Here's how the part is built. I have some questions about the finished solid (model axes, mm). Face numbers are marked on the shaded views. A direction names the side the tool comes from. Round coordinates to 2 decimals unless told otherwise and drop trailing zeros. Order: outer loops, then holes, each group sorted by start corner. A loop starts at its lowest first (then second) coordinate and runs counter-clockwise, first axis right, second up. Notation, with made-up numbers: (80, -20) - (89, -20) arc R28 cw to (89, 5) - close; hole circle Ø1 at (23, -3.5). An arc over 180 degrees is marked (long way). One line per item, written item: value.
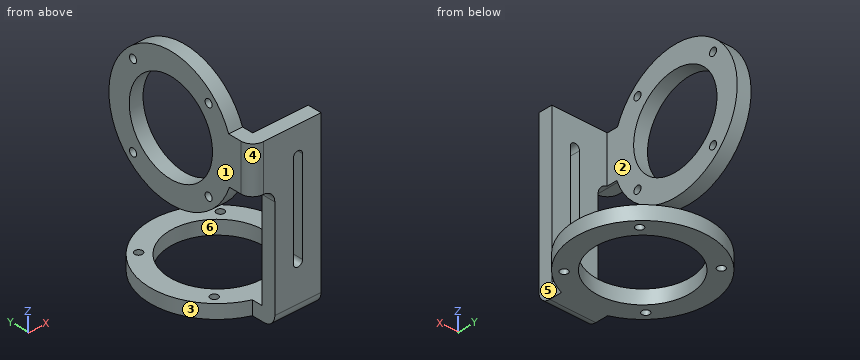
from build123d import *

# Parameters (mm, degrees)
SKETCH1_R           = 29
SKETCH1_R_2         = 20.45
SKETCH1_R_3         = 1.65
BOSS_EXTRUDE1_DEPTH = 6
BOSS_EXTRUDE3_DEPTH = 6
SKETCH4_W           = 20
SKETCH4_H           = 6
BOSS_EXTRUDE4_DEPTH = 67
SKETCH5_W           = 20
SKETCH5_H           = 6
BOSS_EXTRUDE5_DEPTH = 10
SKETCH7_R           = 29
SKETCH7_R_2         = 1.65
SKETCH7_R_3         = 19.5
BOSS_EXTRUDE6_DEPTH = 6
SKETCH8_W           = 6
SKETCH8_H           = 20
BOSS_EXTRUDE8_DEPTH = 6
CUT_EXTRUDE1_DEPTH  = 6
FILLET1_R           = 5
FILLET2_R           = 5


with BuildPart() as part:
    # Sketch1 → Boss-Extrude1 (new body)
    with BuildSketch(Plane.XY):
        Circle(SKETCH1_R)
        Circle(SKETCH1_R_2, mode=Mode.SUBTRACT)
        with Locations((17.68, -17.68)):
            Circle(SKETCH1_R_3, mode=Mode.SUBTRACT)
        with Locations((-17.68, -17.68)):
            Circle(SKETCH1_R_3, mode=Mode.SUBTRACT)
        with Locations((-17.68, 17.68)):
            Circle(SKETCH1_R_3, mode=Mode.SUBTRACT)
        with Locations((17.68, 17.68)):
            Circle(SKETCH1_R_3, mode=Mode.SUBTRACT)
    extrude(amount=BOSS_EXTRUDE1_DEPTH)

    # Sketch3 → Boss-Extrude3 (add)
    with BuildSketch(Plane.XY.offset(6)):
        Polygon((0, -25.748471389), (-10, -25.748471389), (-10, -37.748471389), (10, -37.748471389), (10, -25.748471389), align=None)
    extrude(amount=-BOSS_EXTRUDE3_DEPTH)

    # Sketch4 → Boss-Extrude4 (add)
    with BuildSketch(Plane.XY.offset(6)):
        with Locations((0, -34.748471389)):
            Rectangle(SKETCH4_W, SKETCH4_H)
    extrude(amount=BOSS_EXTRUDE4_DEPTH)

    # Sketch5 → Boss-Extrude5 (add)
    with BuildSketch(Plane.ZY.offset(10)):
        with Locations((63, -34.748471389)):
            Rectangle(SKETCH5_W, SKETCH5_H)
    extrude(amount=BOSS_EXTRUDE5_DEPTH)



with BuildPart() as body_2:
    # Sketch7 → Boss-Extrude6 (new body)
    with BuildSketch(Plane.ZY.offset(20)):
        with Locations(Location((62.50384549, 0.087350514, 0), (0, 0, 270))):
            Circle(SKETCH7_R)
        with Locations(Location((80.18384549, -17.592649486, 0), (0, 0, 270))):
            Circle(SKETCH7_R_2, mode=Mode.SUBTRACT)
        with Locations(Location((44.82384549, -17.592649486, 0), (0, 0, 270))):
            Circle(SKETCH7_R_2, mode=Mode.SUBTRACT)
        with Locations(Location((44.82384549, 17.767350514, 0), (0, 0, 270))):
            Circle(SKETCH7_R_2, mode=Mode.SUBTRACT)
        with Locations(Location((80.18384549, 17.767350514, 0), (0, 0, 270))):
            Circle(SKETCH7_R_2, mode=Mode.SUBTRACT)
        with Locations(Location((62.50384549, 0.087350514, 0), (0, 0, 270))):
            Circle(SKETCH7_R_3, mode=Mode.SUBTRACT)
    extrude(amount=-BOSS_EXTRUDE6_DEPTH)


with BuildPart() as part_1:
    add(part.part)

    add(body_2.part)  # Boss-Extrude8 merges body 2
    # Sketch8 → Boss-Extrude8 (add)
    with BuildSketch(Plane(origin=(0, -31.748471389, 0), x_dir=(1, 0, 0), z_dir=(0, 1, 0))):
        with Locations((-17, -63)):
            Rectangle(SKETCH8_W, SKETCH8_H)
    extrude(amount=BOSS_EXTRUDE8_DEPTH)

    # Sketch9 → Cut-Extrude1 (cut)
    with BuildSketch(Plane.XZ.offset(37.748471389)):
        with BuildLine():
            Line((2, 61), (2, 21))
            ThreePointArc((2, 21), (0, 19), (-2, 21))
            Line((-2, 21), (-2, 61))
            ThreePointArc((-2, 61), (0, 63), (2, 61))
        make_face()
    extrude(amount=-CUT_EXTRUDE1_DEPTH, mode=Mode.SUBTRACT)

    # Fillet1
    fillet1_edges = [part_1.edges().sort_by_distance(p)[0] for p in [
        (0, -37.748471389, 0),
        (-20, -37.748471389, 63),
    ]]
    fillet(fillet1_edges, radius=FILLET1_R)

    # Fillet2
    fillet2_edges = [part_1.edges().sort_by_distance(p)[0] for p in [
        (-10, -34.748471389, 53),
    ]]
    fillet(fillet2_edges, radius=FILLET2_R)


solid = part_1.part
Q1. Will these pins go through, and if not, where does the flat tip stop? pin 1 (4 mm diameter, centred on y = 17.77, z = 80.18, fed in from +X); pin 2 (1.8 mm diameter, centred on y = -35.5, z = 50.5, fed in from +X); pin 3 (12 mm diameter, centred on x = 1.5, z = 31, fed in from +Y).
Results list:
pin 1: x = -14
pin 2: x = 10
pin 3: y = -31.75
Q2. We'd pull the mould along Y, two halves only. Please class the marked faces 4, 5 and 6: released by +Y, released by -Y, zero draft, split by the parting line, or undercut.
Results list:
face 4: released by -Y
face 5: zero draft
face 6: undercut
Q3. If we section it at D-D, the plane y = 0: Please give me the cut outline in (x, z).
Results list:
outline: (-29, 0) - (-20.45, 0) - (-20.45, 6) - (-29, 6) - close; (-20, 33.5) - (-14, 33.5) - (-14, 43) - (-20, 43) - close; (-20, 82) - (-14, 82) - (-14, 91.5) - (-20, 91.5) - close; (20.45, 0) - (29, 0) - (29, 6) - (20.45, 6) - close
Q4. Which directions (+Z, -Z, +X, -X, +Y, -Y) give clear straight access to the entire face, cutting with the end or side of a thin tool? Please do the marked faces 1, 2 and 3.
Results list:
face 1: +Z, -X, +Y, -Y
face 2: +Z, +X, +Y
face 3: -Z
Q5. If we section it at A-A, the plane x = 0: Please give me the cut outline in (y, z).
Results list:
outline: (-37.75, 5) arc R5 ccw to (-32.75, 0) - (-20.45, 0) - (-20.45, 6) - (-31.75, 6) - (-31.75, 19) - (-37.75, 19) - close; (-37.75, 63) - (-31.75, 63) - (-31.75, 73) - (-37.75, 73) - close; (20.45, 0) - (29, 0) - (29, 6) - (20.45, 6) - close
Q6. If we section it at B-B, the plane y = -17.68: Give the number of separate pieces and of enclosed holes in the cut face, then the cut area to 3 significant figures.
Results list:
separate pieces: 8
enclosed holes: 0
area: 252 mm²
Q7. If I drill on line 1 along Z through (x, y) = (6, -24.5); line 2 along Z through (x, y) = (-17, 11); line 3 along Y through (x, z) = (7, 7.5), over which ranges is the centre line in solid material (lowest first)?
Results list:
line 1: 0 to 6
line 2: 35.64 to 46.34, 78.66 to 89.37
line 3: -37.75 to -31.75
Q8. If we section it at C-C, the plane x = 17.68: Please give me the cut outline in (y, z).
Results list:
outline: (-22.99, 0) - (-19.33, 0) - (-19.33, 6) - (-22.99, 6) - close; (-16.03, 0) - (-10.28, 0) - (-10.28, 6) - (-16.03, 6) - close; (10.28, 0) - (16.03, 0) - (16.03, 6) - (10.28, 6) - close; (19.33, 0) - (22.99, 0) - (22.99, 6) - (19.33, 6) - close
